The listing builds one solid part. Answer for the finished solid, in the listing's coordinates (mm). Face numbers are marked on the shaded views. A direction names the side the tool comes from. Give positions to 0.01 mm unless a question says otherwise; leave off trailing zeros. Write each loop counter-clockwise with the first axis right and the second up, starting at its lowest first coordinate (ties: lowest second). Pieces come first, ordered by that corner, then holes.
```python
from build123d import *

# Parameters (mm, degrees)
F0_W      = 40
F0_H      = 35
F1_DEPTH  = 4
F2_W      = 30
F2_H      = 20
F3_DEPTH  = 30
F4_W      = 30
F4_H      = 30
F5_DEPTH  = 10
F6_R      = 1.5
F6_R_2    = 12.5
F7_DEPTH  = 10
F8_R      = 2.5
F9_DEPTH  = 5
F10_W     = 25
F10_H     = 18
F11_DEPTH = 13
F12_R     = 2.5
F13_DEPTH = 5
F14_SIZE  = 2.5


with BuildPart() as f1:
    # F0 (on Top) → F1 (new body)
    with BuildSketch(Plane.XY):
        with Locations((0, 17.5)):
            Rectangle(F0_W, F0_H)
    extrude(amount=F1_DEPTH)



with BuildPart() as f3:
    # F2 (on face) → F3 (new body)
    with BuildSketch(Plane(origin=(0, 0, 0), x_dir=(1, 0, 0), z_dir=(0, 0, -1))):
        with Locations((0, -15)):
            Rectangle(F2_W, F2_H)
    extrude(amount=F3_DEPTH)

    # F8 (on face) → F9 (join)
    with BuildSketch(Plane(origin=(0, 0, -30), x_dir=(1, 0, 0), z_dir=(0, 0, -1))):
        with Locations((-8, -15)):
            Circle(F8_R)
        with Locations((8, -15)):
            Circle(F8_R)
    extrude(amount=F9_DEPTH)

    # F10 (on face) → F11 (join)
    with BuildSketch(Plane(origin=(0, 0, -35), x_dir=(1, 0, 0), z_dir=(0, 0, -1))):
        with Locations((17.5, -20)):
            Rectangle(F10_W, F10_H)
        with Locations((-17.5, -20)):
            Rectangle(F10_W, F10_H)
    extrude(amount=F11_DEPTH)


with BuildPart() as f5:
    # F4 (on face) → F5 (new body)
    with BuildSketch(Plane.XZ.offset(-5)):
        with Locations((0, -15)):
            Rectangle(F4_W, F4_H)
    extrude(amount=F5_DEPTH)

    # F6 (on face) → F7 (cut, through all)
    with BuildSketch(Plane.XZ.offset(5)):
        with Locations((-12.5, -2.5)):
            Circle(F6_R)
        with Locations((0, -15)):
            Circle(F6_R_2)
        with Locations((12.5, -2.5)):
            Circle(F6_R)
        with Locations((-12.5, -27.5)):
            Circle(F6_R)
        with Locations((12.5, -27.5)):
            Circle(F6_R)
    extrude(amount=-F7_DEPTH, mode=Mode.SUBTRACT)


with BuildPart() as f1_1:
    add(f1.part)

    add(f3.part)  # F13 merges F3

    add(f5.part)  # F13 merges F5
    # F12 (on face) → F13 (join)
    with BuildSketch(Plane(origin=(0, 0, -48), x_dir=(1, 0, 0), z_dir=(0, 0, -1))):
        with Locations((8, -15)):
            Circle(F12_R)
        with Locations((-8, -15)):
            Circle(F12_R)
    extrude(amount=F13_DEPTH)

    # F14
    f14_edges = [f1_1.edges().sort_by_distance(p)[0] for p in [
        (-10.5, 15, -53),
        (5.5, 15, -53),
    ]]
    chamfer(f14_edges, length=F14_SIZE)


solid = f1_1.part
```
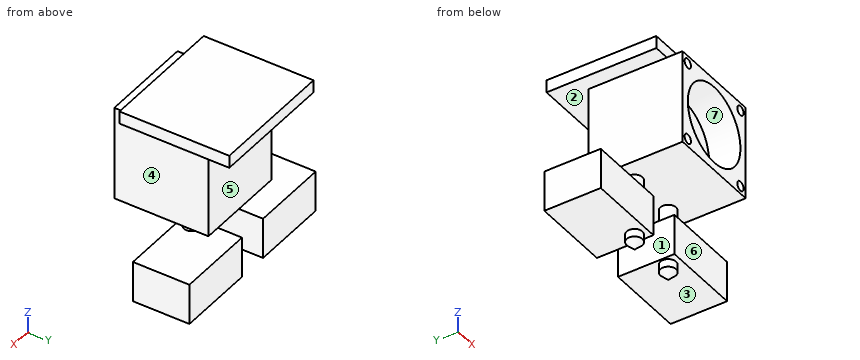
Item 1: A cutting plane is placed at D-D, the plane z = -15. Give the vertices of the cut face in (x, y).
Conclusion:
outline: (-15, -5) - (-12.5, -5) - (-12.5, 5) - (12.5, 5) - (12.5, -5) - (15, -5) - (15, 25) - (-15, 25) - close
Item 2: Each of these flat-tipped pins is pushed along its axis until it touches: P1, Ø20, axis at x = 23, y = 18, coming from the +Z side; P2, Ø3, axis at x = -14, y = 9, coming from the -Z side; P3, Ø2, axis at y = 9.5, z = 1, coming from the -X side; P4, Ø4, axis at x = 20.5, y = 18.5, coming from the -Z side. Where does it stop, or does it pass through?
Conclusion:
P1: stops at z = 4
P2: stops at z = -30
P3: stops at x = -20
P4: stops at z = -48
Item 3: Which of the six approach directions +Z, -Z, +X, -X, +Y, -Y give full straight-line access (tool end or side, diameter ignored) to the marked faces 4, 5, 6 and 7?
Conclusion:
face 4: +X, +Y, -Y
face 5: +X, -X, +Y
face 6: -Z, +X, -X, -Y
face 7: -Y
Item 4: A cutting plane is placed at C-C, the plane y = 20. Give the vertices of the cut face in (x, z), plus the area to 3 significant figures.
Conclusion:
outline: (-30, -48) - (-5, -48) - (-5, -35) - (-30, -35) - close; (-20, 0) - (-15, 0) - (-15, -30) - (15, -30) - (15, 0) - (20, 0) - (20, 4) - (-20, 4) - close; (5, -48) - (30, -48) - (30, -35) - (5, -35) - close
area: 1,710 mm2
Item 5: Determine the mould class of the marked faces 1, 2 and 3 for opening direction Z: pulls with the +Z half, pulls with the -Z half, needs draft (parallel to the pull), parting line crosses it, or undercut.
Conclusion:
face 1: needs draft
face 2: undercut
face 3: pulls with the -Z half
Item 6: A cutting plane is placed at B-B, the plane y = 3.5. Give the vertices of the cut face in (x, z), plus the area to 3 significant figures.
Conclusion:
outline: (-20, 0) - (-15, 0) - (-15, -30) - (15, -30) - (15, 0) - (20, 0) - (20, 4) - (-20, 4) - close; hole circle Ø3 at (-12.5, -27.5); hole circle Ø3 at (-12.5, -2.5); hole circle Ø25 at (0, -15); hole circle Ø3 at (12.5, -27.5); hole circle Ø3 at (12.5, -2.5)
area: 541 mm2
Item 7: Consider probe 1 along X at (y, z) = (23, -39); probe 2 along Z at (x, y) = (14, 18.5); probe 3 along X at (y, z) = (7, -29). Determine where each line is inside the solid, lowest interval first.
Conclusion:
probe 1: x = -30 to -5, 5 to 30
probe 2: z = -48 to -35, -30 to 4
probe 3: x = -15 to 15
Item 8: A cutting plane is placed at A-A, the plane z = -39.5. Give the vertices of the cut face in (x, y), plus the area to 3 significant figures.
Conclusion:
outline: (-30, 11) - (-5, 11) - (-5, 29) - (-30, 29) - close; (5, 11) - (30, 11) - (30, 29) - (5, 29) - close
area: 900 mm2
